from build123d import *

# Parameters (mm, degrees)
BOSS_EXTRUDE1_DEPTH = 70
FILLET2_R           = 1


with BuildPart() as part:
    # Sketch1 → Boss-Extrude1 (new body)
    with BuildSketch(Plane.XY):
        with BuildLine():
            Line((0, 0), (5.5, 0))
            Line((5.5, 0), (5.5, -10))
            ThreePointArc((5.5, -10), (13.263932023, -19.746794345), (24.5, -14.358898944))
            Line((24.5, -14.358898944), (26.5, -14.358898944))
            ThreePointArc((26.5, -14.358898944), (35.5, -20), (44.5, -14.358898944))
            Line((44.5, -14.358898944), (46.5, -14.358898944))
            ThreePointArc((46.5, -14.358898944), (55.5, -20), (64.5, -14.358898944))
            Line((64.5, -14.358898944), (66.5, -14.358898944))
            ThreePointArc((66.5, -14.358898944), (77.736067977, -19.746794345), (85.5, -10))
            Line((85.5, -10), (85.5, 0))
            Line((85.5, 0), (91, 0))
            Line((91, 0), (91, -3))
            Line((91, -3), (87.5, -3))
            Line((87.5, -3), (87.5, -10))
            ThreePointArc((87.5, -10), (80.398979486, -20.95445115), (67.5, -18.94427191))
            Line((67.5, -18.94427191), (63.5, -18.94427191))
            ThreePointArc((63.5, -18.94427191), (55.5, -22), (47.5, -18.94427191))
            Line((47.5, -18.94427191), (43.5, -18.94427191))
            ThreePointArc((43.5, -18.94427191), (35.5, -22), (27.5, -18.94427191))
            Line((27.5, -18.94427191), (23.5, -18.94427191))
            ThreePointArc((23.5, -18.94427191), (10.601020514, -20.95445115), (3.5, -10))
            Line((3.5, -10), (3.5, -3))
            Line((3.5, -3), (0, -3))
            Line((0, -3), (0, 0))
        make_face()
    extrude(amount=BOSS_EXTRUDE1_DEPTH)

    # Fillet2
    fillet2_edges = [part.edges().sort_by_distance(p)[0] for p in [
        (87.5, -3, 35),
        (3.5, -3, 35),
    ]]
    fillet(fillet2_edges, radius=FILLET2_R)


solid = part.part
Geometry check sheet. Reference: the model listing, model coordinates, mm. A direction names the side the tool comes from. Give positions to 0.01 mm unless a question says otherwise; leave off trailing zeros. Loops run counter-clockwise (first coordinate to the right, second up) from the corner with the lowest first, then second, coordinate; pieces in that order, holes last. Notation, with made-up numbers: M -23,15 L 29,15 A22 cw 29,39 Z; hole C 5.25,-12.75 d7. An arc over 180 degrees is marked long. Answer as a JSON object with one key per item and string values. Group by question number.
Item 1: Sectioned sample at C-C on y = -16.25. Record the boundary of the cut face in (x, z).
Item 2: Sectioned sample at A-A on y = -6.75. Record the boundary of the cut face in (x, z), plus the area to 3 significant figures.
Item 3: Sectioned sample at D-D on x = 73.5. Record the boundary of the cut face in (y, z).
Item 4: Material ranges on L1, parallel to X at y = -15.75, z = 63.5; L2, parallel to X at y = -5.25, z = 22; L3, parallel to X at y = -17.5, z = 59, recorded low to high.
Item 5: Gauge pin test, flat ends, axial feed: pin 1 (1 mm diameter, centred on x = 24.5, z = 47.5, fed in from +Y); pin 2 (1 mm diameter, centred on x = 21, z = 16.5, fed in from -Y); pin 3 (4.5 mm diameter, centred on x = 65.5, z = 50.5, fed in from -Y). Record the tip position at first contact, or that the pin passes through.
Item 6: Access from +Z, -Z, +X, -X, +Y, -Y to the whole of each face (thin tool, end or side, straight path). Record for faces 1 (the flat face through (87.5, -7, 35)), 2 (the flat face through (65, -14.359, 35)), 3 (the flat face through (26, -18.944, 35)).
Item 7: Sectioned sample at B-B on z = 23. Record the boundary of the cut face in (x, y), plus the area to 3 significant figures.
Item 8: Mould release check, pull along X, two halves, no side actions. Record for faces 4 (the cylindrical face through (80.575, -20.874, 34.51)), 5 (the flat face through (3.5, -7, 35)), 6 (the flat face through (85.5, -5, 35)), 7 (the flat face through (46, -15, 70)): pulls with the +X half, pulls with the -X half, needs draft (parallel to the pull), parting line crosses it, or undercut.
Findings below:
{
 "1": {"outline": "M 5.26,0 L 7.69,0 L 7.69,70 L 5.26,70 Z; M 23.31,0 L 27.69,0 L 27.69,70 L 23.31,70 Z; M 43.31,0 L 47.69,0 L 47.69,70 L 43.31,70 Z; M 63.31,0 L 67.69,0 L 67.69,70 L 63.31,70 Z; M 83.31,0 L 85.74,0 L 85.74,70 L 83.31,70 Z"},
 "2": {"outline": "M 3.5,0 L 5.5,0 L 5.5,70 L 3.5,70 Z; M 85.5,0 L 87.5,0 L 87.5,70 L 85.5,70 Z", "area": "280 mm2"},
 "3": {"outline": "M -21.83,0 L -19.8,0 L -19.8,70 L -21.83,70 Z"},
 "4": {"L1": "4.97 to 7.32, 23.68 to 27.32, 43.68 to 47.32, 63.68 to 67.32, 83.68 to 86.03", "L2": "3.5 to 5.5, 85.5 to 87.5", "L3": "6.13 to 8.89, 22.11 to 28.89, 42.11 to 48.89, 62.11 to 68.89, 82.11 to 84.87"},
 "5": {"pin 1": "y = -14.36", "pin 2": "y = -20.91", "pin 3": "y = -19.16"},
 "6": {"face 1": "+Z, -Z, +X, -Y", "face 2": "+Z, -Z, +Y", "face 3": "+Z, -Z, -Y"},
 "7": {"outline": "M 0,-3 L 2.5,-3 A1 cw 3.5,-4 L 3.5,-10 A12 ccw 23.5,-18.94 L 27.5,-18.94 A12 ccw 43.5,-18.94 L 47.5,-18.94 A12 ccw 63.5,-18.94 L 67.5,-18.94 A12 ccw 87.5,-10 L 87.5,-4 A1 cw 88.5,-3 L 91,-3 L 91,0 L 85.5,0 L 85.5,-10 A10 cw 66.5,-14.36 L 64.5,-14.36 A10 cw 46.5,-14.36 L 44.5,-14.36 A10 cw 26.5,-14.36 L 24.5,-14.36 A10 cw 5.5,-10 L 5.5,0 L 0,0 Z", "area": "288 mm2"},
 "8": {"face 4": "undercut", "face 5": "pulls with the -X half", "face 6": "undercut", "face 7": "needs draft"}
}
